Can you work these out from the model? Positions are in its coordinate system, mm. A direction names the side the tool comes from. Give positions to 0.01 mm unless a question says otherwise; leave off trailing zeros. Order: outer loops, then holes, each group sorted by start corner. A loop starts at its lowest first (then second) coordinate and runs counter-clockwise, first axis right, second up. Notation, with made-up numbers: M 30,41 L 51,41 A28 cw 51,64 Z; hole C -23,-17 d10. An arc over 180 degrees is marked long. Use one line per item in the form item = value. Start each with the question number.
1. I want a section at C-C, the plane z = -8.5. List the corners of the cut face in (x, y) for me.
2. I want a section at D-D, the plane y = 15.5. List the corners of the cut face in (x, z) for me.
3. I want a section at B-B, the plane z = -50.8. List the corners of the cut face in (x, y) for me, and give its area (3 significant figures).
4. Will these pins go through, and if not, where does the flat tip stop? P1, Ø5, axis at x = 35.5, y = -1, coming from the -Z side; P2, Ø17, axis at x = 3.5, y = 5, coming from the +Z side; P3, Ø8, axis at x = 41, z = -33, coming from the -Y side.
5. I need wall thicknesses on L1, parallel to Y at x = 16, z = -50.5; L2, parallel to Y at x = 1.5, z = -56.5; L3, parallel to Z at x = 13, y = 0. Which ranges of each line are inside material? Lowest first, please.
6. I want a section at A-A, the plane y = 0. List the corners of the cut face in (x, z) for me.
7. For faces 4 (the face through (-20.364, 0.896, -50.089)), 5 (the face through (13.892, 12.592, -49.147)), 6 (the face through (50.8, -17, -48)), 7 (the face through (-3, 13, -31.75)), 8 (the face through (-16, 5.04, -85.95)), which set-ups out of +Z, -Z, +X, -X, +Y, -Y let a thin tool reach every point of the face, with its end or its side?
8. We'd pull the mould along Z, two halves only. Please class faces 1 (the face through (31.4, -16.18, -63.2)), 2 (the face through (-17, -3, -101.6)), 3 (the face through (35.15, 5.04, -66.8)): +Z half, -Z half, draft (parallel to the pull), parting line (faces both ways), or undercut.
Autodesk Inventor part; units mm, degrees
ref_plane "Work Plane1" through (20.3835, 0, 0) normal (-1, 0, 0) x (0, 1, 0)
ref_plane "YZ Plane" through (0, 0, 0) normal (1, 0, 0) x (0, 1, 0)
ref_plane "XZ Plane" through (0, 0, 0) normal (0, 1, 0) x (-1, 0, 0)
sketch "Sketch1" plane through (0, 0, 0) normal (0, 0, 1) x (1, 0, 0)
  circle A0 centre (0, 0) radius 20.3835
  dimension "d0" = 40.767
extrude "Extrusion1" add sketch "Sketch1" against normal blind 101.6
sketch "Sketch2" plane through (0, 0, 0) normal (0, 0, 1) x (1, 0, 0)
  circle A0 centre (0, 0) radius 20.3835
  line L0 (20.3835, 0) -> (20.3835, 20.3835)
sketch "Sketch3" plane through (0, 0, -101.6) normal (0, 0, -1) x (-1, 0, 0)
  circle A0 centre (0, 0) radius 20.3835
  line L0 (-20.3835, 0) -> (-20.3835, 20.3835)
ref_plane "Work Plane1" through (20.3835, 0, 0) normal (-1, 0, 0) x (0, 1, 0)
sketch "Sketch4" plane through (20.3835, 0, 0) normal (-1, 0, 0) x (0, 1, 0)
  line L0 (20.3835, 101.6) -> (-20.3835, 101.6)
  circle A0 centre (0, 50.8) radius 20.3835
  line L1 (-20.3835, 0) -> (-20.3835, 101.6)
  point P0 (0, 0)
extrude "Extrusion2" add sketch "Sketch4" against normal blind 30.4165
extrude "Extrusion3" add sketch "Sketch4" along normal blind 20.3835
sketch "Sketch5" plane through (0, 0, 0) normal (0, 0, 1) x (1, 0, 0)
  circle A0 centre (0, 0) radius 16.7767
  dimension "d7" = 33.5534
sketch "Sketch6" plane through (0, 0, 0) normal (0, 0, 1) x (1, 0, 0)
  circle A0 centre (0, 0) radius 12.7
  dimension "d8" = 25.4
sketch "Sketch7" plane through (50.8, 0, -50.8) normal (1, 0, 0) x (0, 0, -1)
  circle A0 centre (0, 0) radius 16.7767
  point P0 (-50.8, 0)
  dimension "d9" = 33.5534
sketch "Sketch8" plane through (50.8, 0, -50.8) normal (1, 0, 0) x (0, 0, -1)
  circle A0 centre (0, 0) radius 12.7
  point P0 (-50.8, 0)
  dimension "d10" = 25.4
sketch "Sketch9" plane through (0, 0, -101.6) normal (0, 0, -1) x (-1, 0, 0)
  circle A0 centre (0, 0) radius 16.7767
  dimension "d11" = 33.5534
extrude "Extrusion4" cut sketch "Sketch9" against normal blind 31.75
extrude "Extrusion5" cut sketch "Sketch7" against normal blind 31.75
extrude "Extrusion6" cut sketch "Sketch5" against normal blind 31.75
extrude "Extrusion7" cut sketch "Sketch6" against normal blind 101.6
extrude "Extrusion8" cut sketch "Sketch8" against normal blind 50.8
properties part number "Tee 1 Inch"
Check result:
q1.outline = C 0,0 d40.77; hole C 0,0 d33.55
q2.outline = M -13.24,-101.6 L -6.42,-101.6 L -6.42,-69.85 L 6.42,-69.85 L 6.42,-101.6 L 13.24,-101.6 L 13.24,-64.04 L 50.8,-64.04 L 50.8,-57.22 L 19.05,-57.22 L 19.05,-44.38 L 50.8,-44.38 L 50.8,-37.56 L 13.24,-37.56 L 13.24,0 L 6.42,0 L 6.42,-31.75 L -6.42,-31.75 L -6.42,0 L -13.24,0 Z
q3.outline = M 0,-20.38 L 50.8,-20.38 L 50.8,-16.78 L 19.05,-16.78 L 19.05,-12.7 L 0,-12.7 A12.7 cw 0,12.7 L 19.05,12.7 L 19.05,16.78 L 50.8,16.78 L 50.8,20.38 L 0,20.38 A20.38 ccw Z
q3.area = 921 mm2
q4.P1 = -71.18
q4.P2 = -31.75
q4.P3 = -15
q5.L1 = -20.38 to -12.7, 12.7 to 20.38
q5.L2 = -20.33 to -12.61, 12.61 to 20.33
q5.L3 = -69.85 to -63.5, -38.1 to -31.75
q6.outline = M -20.38,-101.6 L -16.78,-101.6 L -16.78,-69.85 L -12.7,-69.85 L -12.7,-31.75 L -16.78,-31.75 L -16.78,0 L -20.38,0 Z; M 12.7,-69.85 L 16.78,-69.85 L 16.78,-101.6 L 20.38,-101.6 L 20.38,-71.18 L 50.8,-71.18 L 50.8,-67.58 L 19.05,-67.58 L 19.05,-63.5 L 12.7,-63.5 Z; M 12.7,-38.1 L 19.05,-38.1 L 19.05,-34.02 L 50.8,-34.02 L 50.8,-30.42 L 20.38,-30.42 L 20.38,0 L 16.78,0 L 16.78,-31.75 L 12.7,-31.75 Z
q7.face_4 = none
q7.face_5 = +X
q7.face_6 = +Z, -Z, +X, +Y, -Y
q7.face_7 = +Z
q7.face_8 = -Z
q8.face_1 = parting line
q8.face_2 = -Z half
q8.face_3 = undercut
